from build123d import *

# Parameters (mm, degrees)
BOSS_EXTRUDE1_DEPTH = 75
SKETCH2_W           = 15.96
SKETCH2_H           = 40
CUT_EXTRUDE1_DEPTH  = 5


with BuildPart() as part:
    # Sketch1 → Boss-Extrude1 (new body)
    with BuildSketch(Plane(origin=(0, 0, 0), x_dir=(0, 0, -1), z_dir=(1, 0, 0))):
        Polygon((65, -12.06), (-65, -12.06), (-65, 13.823269807), (-54.438417974, 42.840977937), (-45.040373426, 39.423849117), (-55, 12.06), (65, 12.06), align=None)
    extrude(amount=-BOSS_EXTRUDE1_DEPTH)

    # Sketch2 → Cut-Extrude1 (cut)
    with BuildSketch(Plane(origin=(0, 22.507612708, 61.83915768), x_dir=(1, 0, 0), z_dir=(0, 0.342020143325673, 0.9396926207859068))):
        with Locations((-36.611821511, 9.548315317)):
            Rectangle(SKETCH2_W, SKETCH2_H)
    extrude(amount=-CUT_EXTRUDE1_DEPTH, mode=Mode.SUBTRACT)


solid = part.part
The listing builds one solid part. Answer for the finished solid, in the listing's coordinates (mm). A direction names the side the tool comes from. Round coordinates to 2 decimals unless told otherwise and drop trailing zeros. Order: outer loops, then holes, each group sorted by start corner. A loop starts at its lowest first (then second) coordinate and runs counter-clockwise, first axis right, second up. Notation, with made-up numbers: (19.25, 30) -> (49.25, 30) arc R17 ccw to (49.25, 50) -> close; hole circle Ø7 at (79, 58). An arc over 180 degrees is marked (long way). Write each question's results on one line, items separated by ' | '. Start each with the question number.
Q1. Find section A-A (x = -32). Determine the outline of the cut face in (y, z), then the cut area to 3 significant figures.
Q2. Find section B-B (y = 21). Determine the outline of the cut face in (x, z), then the cut area to 3 significant figures.
Q3. Each of these flat-tipped pins is pushed along its axis until it touches: pin 1 (3 mm diameter, centred on x = -67.5, y = 34.5, fed in from +Z); pin 2 (2 mm diameter, centred on x = -25, y = 16, fed in from -Z); pin 3 (6 mm diameter, centred on x = -64.5, y = 37, fed in from -Z). Where does it stop, or does it pass through?
Q4. Straight lines are drawn through the part: probe 1 along Y at (x, z) = (-41.5, 4.5); probe 2 along Z at (x, y) = (-22, 20.5); probe 3 along Z at (x, y) = (-24, 23.5). For each, find the intervals that lie inside material, in ascending order. Write a range as from..to.
Q5. Which of the six approach directions +Z, -Z, +X, -X, +Y, -Y give full straight-line access (tool end or side, diameter ignored) to faces 1 (the flat face through (-36.98, 25.93, 49.95)), 2 (the flat face through (-36.975, 40.777, 48.761)), 3 (the flat face through (-36.724, 11.767, 62.888))?
Q6. Find section C-C (z = -50.5). Determine the outline of the cut face in (x, y).
Q7. Find section D-D (x = -11). Determine the outline of the cut face in (y, z), then the cut area to 3 significant figures.
Q8. The mould has two halves that part along X. Classify faces 4 (the flat face through (0, 4, -1)), 5 (the flat face through (-14.115, 28.129, 59.793)), 6 (the flat face through (-28.632, 27, 58)): pulls with the +X half, pulls with the -X half, needs draft (parallel to the pull), parting line crosses it, or undercut.
Worked answers:
1) outline: (-12.06, -65) -> (12.06, -65) -> (12.06, 55) -> (39.42, 45.04) -> (41.13, 49.74) -> (10.98, 60.72) -> (12.54, 65) -> (-12.06, 65) -> close | area: 3,280 mm2
2) outline: (-75, 51.75) -> (0, 51.75) -> (0, 62.39) -> (-28.63, 62.39) -> (-28.63, 57.07) -> (-44.59, 57.07) -> (-44.59, 62.39) -> (-75, 62.39) -> close | area: 713 mm2
3) pin 1: stops at z = 58.02 | pin 2: stops at z = 53.2 | pin 3: stops at z = 45.04
4) probe 1: y = -12.06..12.06 | probe 2: z = 51.93..62.57 | probe 3: z = 50.84..61.48
5) face 1: -Z, +X, -X | face 2: -Z, +X, -X, +Y | face 3: +Y
6) outline: (-75, -12.06) -> (0, -12.06) -> (0, 12.06) -> (-75, 12.06) -> close
7) outline: (-12.06, -65) -> (12.06, -65) -> (12.06, 55) -> (39.42, 45.04) -> (42.84, 54.44) -> (13.82, 65) -> (-12.06, 65) -> close | area: 3,440 mm2
8) face 4: pulls with the +X half | face 5: needs draft | face 6: undercut
